Could you check a few things on this model? Use its own coordinates, in mm. A direction names the side the tool comes from. Coordinates: 2 decimals unless noted, no trailing zeros. Loops run counter-clockwise (first coordinate to the right, second up) from the corner with the lowest first, then second, coordinate; pieces in that order, holes last. Notation, with made-up numbers: (37.25, 21.25) -> (82.25, 21.25) arc R30 cw to (82.25, 43.25) -> close; hole circle Ø2 at (-36.5, -29.5). An arc over 180 degrees is marked (long way). One line per question, with ' | ' between items.
from build123d import *

# Parameters (mm, degrees)
SKETCH1_W           = 136
SKETCH1_H           = 46
SKETCH1_R           = 1.05
SKETCH1_R_2         = 1.55
BOSS_EXTRUDE1_DEPTH = 3
CUT_EXTRUDE1_REACH  = 5
SKETCH2_W           = 11
SKETCH2_H           = 3
SKETCH2_W_2         = 10
SKETCH2_W_3         = 3
SKETCH2_H_2         = 9
SKETCH2_H_3         = 7


with BuildPart() as part:
    # Sketch1 → Boss-Extrude1 (new body)
    with BuildSketch(Plane.XY):
        with Locations((-68, 23)):
            Rectangle(SKETCH1_W, SKETCH1_H)
        with Locations((-88, 15.95)):
            Circle(SKETCH1_R, mode=Mode.SUBTRACT)
        with Locations((-125.5, 17.25)):
            Circle(SKETCH1_R_2, mode=Mode.SUBTRACT)
        with Locations((-48, 15.95)):
            Circle(SKETCH1_R, mode=Mode.SUBTRACT)
        with Locations((-10.5, 17.25)):
            Circle(SKETCH1_R_2, mode=Mode.SUBTRACT)
    extrude(amount=BOSS_EXTRUDE1_DEPTH)

    # Sketch2 → Cut-Extrude1 (cut, up to next)
    with BuildSketch(Plane.XY.offset(3), mode=Mode.PRIVATE) as cut_extrude1_sk1:
        with Locations((-65.5, 44.5)):
            Rectangle(SKETCH2_W, SKETCH2_H)
    cut_extrude1_tool1 = extrude(cut_extrude1_sk1.sketch, amount=-CUT_EXTRUDE1_REACH, mode=Mode.PRIVATE) & part.part
    add(cut_extrude1_tool1.solids().sort_by_distance((-65.5, 44.5, 3))[0], mode=Mode.SUBTRACT)
    # Sketch2 → Cut-Extrude1 (cut, up to next)
    with BuildSketch(Plane.XY.offset(3), mode=Mode.PRIVATE) as cut_extrude1_sk2:
        with Locations((-91, 44.5)):
            Rectangle(SKETCH2_W_2, SKETCH2_H)
    cut_extrude1_tool2 = extrude(cut_extrude1_sk2.sketch, amount=-CUT_EXTRUDE1_REACH, mode=Mode.PRIVATE) & part.part
    add(cut_extrude1_tool2.solids().sort_by_distance((-91, 44.5, 3))[0], mode=Mode.SUBTRACT)
    # Sketch2 → Cut-Extrude1 (cut, up to next)
    with BuildSketch(Plane.XY.offset(3), mode=Mode.PRIVATE) as cut_extrude1_sk3:
        with Locations((-111, 44.5)):
            Rectangle(SKETCH2_W_2, SKETCH2_H)
    cut_extrude1_tool3 = extrude(cut_extrude1_sk3.sketch, amount=-CUT_EXTRUDE1_REACH, mode=Mode.PRIVATE) & part.part
    add(cut_extrude1_tool3.solids().sort_by_distance((-111, 44.5, 3))[0], mode=Mode.SUBTRACT)
    # Sketch2 → Cut-Extrude1 (cut, up to next)
    with BuildSketch(Plane.XY.offset(3), mode=Mode.PRIVATE) as cut_extrude1_sk4:
        Polygon((-136, 43), (-133, 43), (-126, 43), (-126, 46), (-136, 46), align=None)
    cut_extrude1_tool4 = extrude(cut_extrude1_sk4.sketch, amount=-CUT_EXTRUDE1_REACH, mode=Mode.PRIVATE) & part.part
    add(cut_extrude1_tool4.solids().sort_by_distance((-131, 44.5, 3))[0], mode=Mode.SUBTRACT)
    # Sketch2 → Cut-Extrude1 (cut, up to next)
    with BuildSketch(Plane.XY.offset(3), mode=Mode.PRIVATE) as cut_extrude1_sk5:
        with Locations((-134.5, 38.5)):
            Rectangle(SKETCH2_W_3, SKETCH2_H_2)
    cut_extrude1_tool5 = extrude(cut_extrude1_sk5.sketch, amount=-CUT_EXTRUDE1_REACH, mode=Mode.PRIVATE) & part.part
    add(cut_extrude1_tool5.solids().sort_by_distance((-134.5, 38.5, 3))[0], mode=Mode.SUBTRACT)
    # Sketch2 → Cut-Extrude1 (cut, up to next)
    with BuildSketch(Plane.XY.offset(3), mode=Mode.PRIVATE) as cut_extrude1_sk6:
        with Locations((-134.5, 20.5)):
            Rectangle(SKETCH2_W_3, SKETCH2_H_2)
    cut_extrude1_tool6 = extrude(cut_extrude1_sk6.sketch, amount=-CUT_EXTRUDE1_REACH, mode=Mode.PRIVATE) & part.part
    add(cut_extrude1_tool6.solids().sort_by_distance((-134.5, 20.5, 3))[0], mode=Mode.SUBTRACT)
    # Sketch2 → Cut-Extrude1 (cut, up to next)
    with BuildSketch(Plane.XY.offset(3), mode=Mode.PRIVATE) as cut_extrude1_sk7:
        with Locations((-134.5, 3.5)):
            Rectangle(SKETCH2_W_3, SKETCH2_H_3)
    cut_extrude1_tool7 = extrude(cut_extrude1_sk7.sketch, amount=-CUT_EXTRUDE1_REACH, mode=Mode.PRIVATE) & part.part
    add(cut_extrude1_tool7.solids().sort_by_distance((-134.5, 3.5, 3))[0], mode=Mode.SUBTRACT)
    # Sketch2 → Cut-Extrude1 (cut, up to next)
    with BuildSketch(Plane.XY.offset(3), mode=Mode.PRIVATE) as cut_extrude1_sk8:
        with Locations((-1.5, 3.5)):
            Rectangle(SKETCH2_W_3, SKETCH2_H_3)
    cut_extrude1_tool8 = extrude(cut_extrude1_sk8.sketch, amount=-CUT_EXTRUDE1_REACH, mode=Mode.PRIVATE) & part.part
    add(cut_extrude1_tool8.solids().sort_by_distance((-1.5, 3.5, 3))[0], mode=Mode.SUBTRACT)
    # Sketch2 → Cut-Extrude1 (cut, up to next)
    with BuildSketch(Plane.XY.offset(3), mode=Mode.PRIVATE) as cut_extrude1_sk9:
        with Locations((-1.5, 20.5)):
            Rectangle(SKETCH2_W_3, SKETCH2_H_2)
    cut_extrude1_tool9 = extrude(cut_extrude1_sk9.sketch, amount=-CUT_EXTRUDE1_REACH, mode=Mode.PRIVATE) & part.part
    add(cut_extrude1_tool9.solids().sort_by_distance((-1.5, 20.5, 3))[0], mode=Mode.SUBTRACT)
    # Sketch2 → Cut-Extrude1 (cut, up to next)
    with BuildSketch(Plane.XY.offset(3), mode=Mode.PRIVATE) as cut_extrude1_sk10:
        with Locations((-1.5, 38.5)):
            Rectangle(SKETCH2_W_3, SKETCH2_H_2)
    cut_extrude1_tool10 = extrude(cut_extrude1_sk10.sketch, amount=-CUT_EXTRUDE1_REACH, mode=Mode.PRIVATE) & part.part
    add(cut_extrude1_tool10.solids().sort_by_distance((-1.5, 38.5, 3))[0], mode=Mode.SUBTRACT)
    # Sketch2 → Cut-Extrude1 (cut, up to next)
    with BuildSketch(Plane.XY.offset(3), mode=Mode.PRIVATE) as cut_extrude1_sk11:
        Polygon((0, 46), (-10, 46), (-10, 43), (-3, 43), (0, 43), align=None)
    cut_extrude1_tool11 = extrude(cut_extrude1_sk11.sketch, amount=-CUT_EXTRUDE1_REACH, mode=Mode.PRIVATE) & part.part
    add(cut_extrude1_tool11.solids().sort_by_distance((-5, 44.5, 3))[0], mode=Mode.SUBTRACT)
    # Sketch2 → Cut-Extrude1 (cut, up to next)
    with BuildSketch(Plane.XY.offset(3), mode=Mode.PRIVATE) as cut_extrude1_sk12:
        with Locations((-25, 44.5)):
            Rectangle(SKETCH2_W_2, SKETCH2_H)
    cut_extrude1_tool12 = extrude(cut_extrude1_sk12.sketch, amount=-CUT_EXTRUDE1_REACH, mode=Mode.PRIVATE) & part.part
    add(cut_extrude1_tool12.solids().sort_by_distance((-25, 44.5, 3))[0], mode=Mode.SUBTRACT)
    # Sketch2 → Cut-Extrude1 (cut, up to next)
    with BuildSketch(Plane.XY.offset(3), mode=Mode.PRIVATE) as cut_extrude1_sk13:
        with Locations((-45, 44.5)):
            Rectangle(SKETCH2_W_2, SKETCH2_H)
    cut_extrude1_tool13 = extrude(cut_extrude1_sk13.sketch, amount=-CUT_EXTRUDE1_REACH, mode=Mode.PRIVATE) & part.part
    add(cut_extrude1_tool13.solids().sort_by_distance((-45, 44.5, 3))[0], mode=Mode.SUBTRACT)


solid = part.part
1) I'm going to push flat-ended pins straight in: pin 1 Ø0.9 at (y, z) = (39, 1) entering from +X; pin 2 Ø1.5 at (y, z) = (44, 2) entering from +X; pin 3 Ø1.5 at (y, z) = (44, 1) entering from -X. Where does each tip first touch, or does it pass through?
Data:
pin 1: x = -3 | pin 2: x = -10 | pin 3: x = -126
2) On a 3-axis mill with a long thin cutter (end or side, diameter ignored), from which of +Z, -Z, +X, -X, +Y, -Y can I reach the whole of each face in a straight line? I mean faces 4 (the face through (-111, 43, 2)), 5 (the face through (-2, 7, 2)), 6 (the face through (-2, 16, 2)). Say none if no direction works.
Data:
face 4: +Z, -Z, +Y | face 5: +Z, -Z, +X, -Y | face 6: +Z, -Z, +X
3) If we section it at B-B on x = -110: Please give me the cut outline in (y, z), and give its area (3 significant figures).
Data:
outline: (0, 0) -> (43, 0) -> (43, 3) -> (0, 3) -> close | area: 129 mm²
4) I need wall thicknesses on line 1 along Y through (x, z) = (-48, 2.4); line 2 along Y through (x, z) = (-125.5, 2.15); line 3 along Y through (x, z) = (-8.5, 1.25). Which ranges of each line are inside material? Lowest first, please. Write a range as from..to.
Data:
line 1: 0..14.9, 17..43 | line 2: 0..15.7, 18.8..46 | line 3: 0..43
5) If we section it at C-C on y = 20.5: Please give me the cut outline in (x, z), and give its area (3 significant figures).
Data:
outline: (-133, 0) -> (-3, 0) -> (-3, 3) -> (-133, 3) -> close | area: 390 mm²
6) We'd pull the mould along X, two halves only. Please class faces 1 (the face through (-10, 45, 2)), 2 (the face through (-96, 44, 2)), 3 (the face through (-135, 34, 2)): pulls with the +X half, pulls with the -X half, needs draft (parallel to the pull), parting line crosses it, or undercut.
Data:
face 1: pulls with the +X half | face 2: undercut | face 3: needs draft
7) If we section it at A-A on z = 2.5: Give the number of separate pieces and of enclosed holes in the cut face, and give its area (3 significant figures).
Data:
separate pieces: 1 | enclosed holes: 4 | area: 5,870 mm²
